```python
from build123d import *

# Parameters (mm, degrees)
F0_R     = 4.7625
F1_DEPTH = 1.5875
F2_R     = 3.96875
F3_DEPTH = 8.89
F4_W     = 9.525
F4_H     = 9.525
F5_DEPTH = 19.05
F6_SIZE  = 0.79375
F7_R     = 1.7272
F8_DEPTH = 9.525


with BuildPart() as f1:
    # F0 (on Top) → F1 (new body)
    with BuildSketch(Plane.XY):
        Circle(F0_R)
    extrude(amount=F1_DEPTH)

    # F2 (on face) → F3 (join)
    with BuildSketch(Plane.XY.offset(1.5875)):
        Circle(F2_R)
    extrude(amount=F3_DEPTH)

    # F4 (on face) → F5 (join)
    with BuildSketch(Plane(origin=(0, 0, 0), x_dir=(1, 0, 0), z_dir=(0, 0, -1))):
        Rectangle(F4_W, F4_H)
    extrude(amount=F5_DEPTH)

    # F6
    f6_edges = [f1.edges().sort_by_distance(p)[0] for p in [
        (-3.96875, 0, 10.4775),
    ]]
    chamfer(f6_edges, length=F6_SIZE)

    # F7 (on face) → F8 (cut, through all)
    with BuildSketch(Plane(origin=(0, 4.7625, 0), x_dir=(-1, 0, 0), z_dir=(0, 1, 0))):
        with Locations((0, -4.7625)):
            Circle(F7_R)
        with Locations((0, -14.2875)):
            Circle(F7_R)
    extrude(amount=-F8_DEPTH, mode=Mode.SUBTRACT)


solid = f1.part
```
The listing builds one solid part. Answer for the finished solid, in the listing's coordinates (mm). A direction names the side the tool comes from. Give positions to 0.01 mm unless a question says otherwise; leave off trailing zeros. Order: outer loops, then holes, each group sorted by start corner. A loop starts at its lowest first (then second) coordinate and runs counter-clockwise, first axis right, second up. Notation, with made-up numbers: (0, 36) -> (56, 36) arc R23 ccw to (56, 65) -> close; hole circle Ø3 at (18.25, -4.5). An arc over 180 degrees is marked (long way). Write each question's results on one line, items separated by ' | '.
Q1. The part is cut by section A-A, the plane z = -15.25. Give the vertices of the cut face in (x, y).
Checked values:
outline: (-4.76, -4.76) -> (-1.43, -4.76) -> (-1.43, 4.76) -> (-4.76, 4.76) -> close; (1.43, -4.76) -> (4.76, -4.76) -> (4.76, 4.76) -> (1.43, 4.76) -> close
Q2. Each of these flat-tipped pins is pushed along its axis until it touches: P1, Ø2, axis at y = 0, z = 6, coming from the -X side; P2, Ø1.4, axis at x = 2.5, y = 3, coming from the +Z side. Where does it stop, or does it pass through?
Checked values:
P1: stops at x = -3.97 | P2: stops at z = 10.45
Q3. The part is cut by section B-B, the plane x = 1. State how many separate pieces and enclosed holes the cut face has, and give its area (3 significant figures).
Checked values:
separate pieces: 3 | enclosed holes: 0 | area: 210 mm^2
Q4. Which of the six approach directions +Z, -Z, +X, -X, +Y, -Y give full straight-line access (tool end or side, diameter ignored) to faces 5 (the face through (-4, 4, 0)), 6 (the face through (4, 4, 0)), 7 (the face through (-2, 4, 1.588)), 8 (the face through (-4, -4, 0))?
Checked values:
face 5: +Z, -X, +Y | face 6: +Z, +X, +Y | face 7: +Z | face 8: +Z, -X, -Y
Q5. Determine the mould class of faces 1 (the face through (0.374, 0.067, -15.974)), 2 (the face through (0, -4.762, -9)), 3 (the face through (0, 0, -19.05)), 4 (the face through (4, -4, 0)) for opening direction Z: pulls with the +Z half, pulls with the -Z half, needs draft (parallel to the pull), parting line crosses it, or undercut.
Checked values:
face 1: undercut | face 2: needs draft | face 3: pulls with the -Z half | face 4: pulls with the +Z half
Q6. Straight lines are drawn through the part: probe 1 along Z at (x, y) = (0, 2.75); probe 2 along X at (y, z) = (3.75, -4.75); probe 3 along Z at (x, y) = (0.25, -3.75). For each, find the intervals that lie inside material, in ascending order. Write a range as from..to.
Checked values:
probe 1: z = -19.05..-16.01, -12.56..-6.49, -3.04..10.48 | probe 2: x = -4.76..-1.73, 1.73..4.76 | probe 3: z = -19.05..-16, -12.58..-6.47, -3.05..9.89
